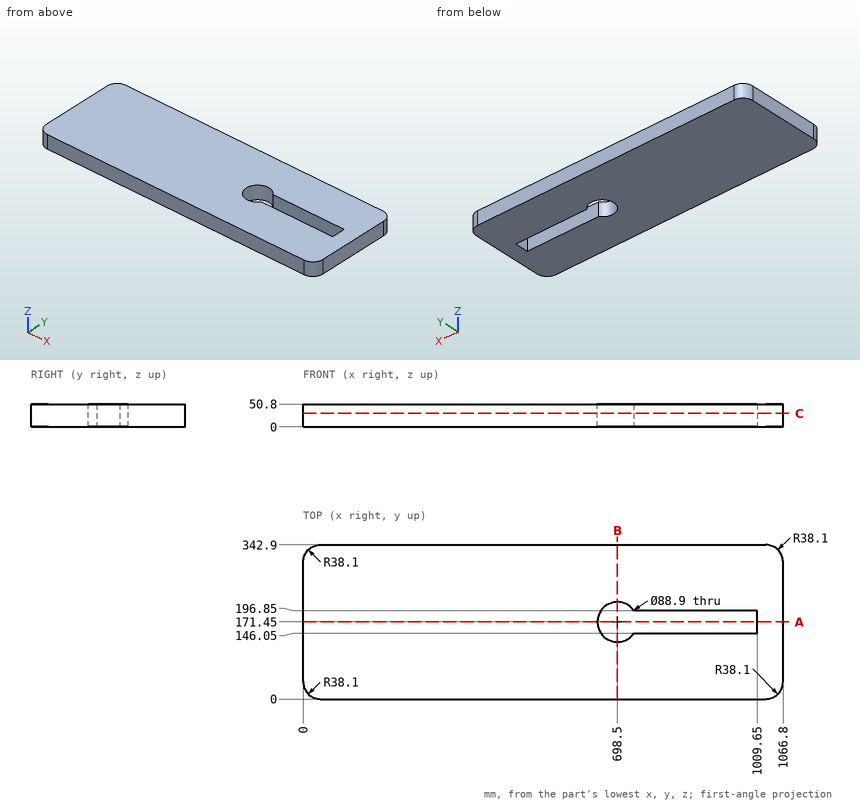
Can you work these out from the drawing? Everything is in mm from the part's minimum corner. Give positions to 0.01 mm unless a question says otherwise; leave off trailing zeros. Loops run counter-clockwise (first coordinate to the right, second up) from the corner with the lowest first, then second, coordinate; pieces in that order, holes last. Notation, with made-up numbers: (66.5, -2.75) - (90.5, -2.75) arc R27 cw to (90.5, 23.25) - close; hole circle Ø2 at (82, 85). An arc over 180 degrees is marked (long way). Answer as a JSON object with one key per item and string values.
Q1. Will this pin go through, and if not, where does the flat tip stop? P1, Ø12, axis at x = 805, z = 41.5, coming from the -Y side.
Geometry says:
{"P1": "y = 0"}
Q2. Imagine slicing it at B-B on x = 698.5. Write out the boundary of the cut face in (y, z), plus the area to 3 significant figures.
Geometry says:
{"outline": "(0, 0) - (127, 0) - (127, 50.8) - (0, 50.8) - close; (215.9, 0) - (342.9, 0) - (342.9, 50.8) - (215.9, 50.8) - close", "area": "12,900 mm²"}
Q3. Imagine slicing it at C-C on z = 30. Write out the boundary of the cut face in (x, y).
Geometry says:
{"outline": "(0, 38.1) arc R38.1 ccw to (38.1, 0) - (1028.7, 0) arc R38.1 ccw to (1066.8, 38.1) - (1066.8, 304.8) arc R38.1 ccw to (1028.7, 342.9) - (38.1, 342.9) arc R38.1 ccw to (0, 304.8) - close; hole (734.98, 146.05) - (1009.65, 146.05) - (1009.65, 196.85) - (734.98, 196.85) arc R44.45 ccw (long way) to start"}
Q4. If I drill on L1, parallel to Y at x = 698.5, z = 38; L2, parallel to X at y = 171.45, z = 22.5; L3, parallel to Y at x = 892, z = 38.5, over which ranges is the centre line in solid material (lowest first)?
Geometry says:
{"L1": "0 to 127, 215.9 to 342.9", "L2": "0 to 654.05, 1009.65 to 1066.8", "L3": "0 to 146.05, 196.85 to 342.9"}
Q5. Imagine slicing it at A-A on y = 171.45. Write out the boundary of the cut face in (x, z).
Geometry says:
{"outline": "(0, 0) - (654.05, 0) - (654.05, 50.8) - (0, 50.8) - close; (1009.65, 0) - (1066.8, 0) - (1066.8, 50.8) - (1009.65, 50.8) - close"}
